The listing builds one solid part. Answer for the finished solid, in the listing's coordinates (mm). A direction names the side the tool comes from. Round coordinates to 2 decimals unless told otherwise and drop trailing zeros. Write each loop counter-clockwise with the first axis right and the second up, starting at its lowest first coordinate (ties: lowest second). Pieces come first, ordered by that corner, then holes.
Item 1: Find the intervals of material crossed by probe 1 along Y at (x, z) = (0, -4.3); probe 2 along X at (y, z) = (-2.6, -3.5); probe 3 along X at (y, z) = (2.5, 0.75), in increasing order.
Item 2: For a pull along X with two mould halves and no side action, classify faces 4 (the face through (0, 26, 5)), 5 (the face through (-6, 26, 0)), 6 (the face through (0, -2, -3.6)) as +X half, -X half, draft (parallel to the pull), parting line (faces both ways), or undercut.
Item 3: Find section B-B on x = 1.25. Give the vertices of the cut face in (y, z).
Item 4: Find section C-C on y = 43. Give the vertices of the cut face in (x, z), then the cut area to 3 significant figures.
Item 5: Find section A-A on z = 1. Give the vertices of the cut face in (x, y).
Item 6: A tool of negligible diameter and unlimited length cuts with its end or side. For faces 1 (the face through (0, 26, -5)), 2 (the face through (-2.7, 53.5, 0)), 3 (the face through (0, -2, 3.6)), from which of +Z, -Z, +X, -X, +Y, -Y can it reach the whole face along a straight path? Write none if from no direction.
```python
from build123d import *

# Parameters (mm, degrees)
SKETCH_1_W          = 12
SKETCH_1_H          = 10
SKETCH_1_W_2        = 6.2
SKETCH_1_H_2        = 6.2
EXTRUDE_1_DEPTH     = 54
EXTRUDE_START       = 54
SKETCH_1_3_W        = 12
SKETCH_1_3_H        = 10
SKETCH_1_3_W_2      = 6.2
SKETCH_1_3_H_2      = 6.2
SKETCH_1_3_W_3      = 5.4
SKETCH_1_3_H_3      = 5.4
EXTRUDE_2_DEPTH     = 1
SKETCH_3_W          = 12
SKETCH_3_H          = 10
SKETCH_3_W_2        = 7.2
SKETCH_3_H_2        = 7.2
EXTRUDE_3_DEPTH     = 3.4
SKETCH_2_R          = 0.3
CUT_EXTRUDE_1_DEPTH = 2
SKETCH_7_R          = 0.3
CUT_EXTRUDE_2_DEPTH = 56.244909268


with BuildPart() as part:
    # 草图1 → 凸台-拉伸1 (new body)
    with BuildSketch(Plane(origin=(0, 0, 0), x_dir=(1, 0, 0), z_dir=(0, 1, 0))):
        Rectangle(SKETCH_1_W, SKETCH_1_H)
        Rectangle(SKETCH_1_W_2, SKETCH_1_H_2, mode=Mode.SUBTRACT)
    extrude(amount=EXTRUDE_1_DEPTH)

    # 草图1<3> → 凸台-拉伸2 (add)
    # profile 1 of 2: a face of its own
    with BuildSketch(Plane(origin=(0, 0, 0), x_dir=(1, 0, 0), z_dir=(0, 1, 0)).offset(EXTRUDE_START)):
        Rectangle(SKETCH_1_3_W, SKETCH_1_3_H)
        Rectangle(SKETCH_1_3_W_2, SKETCH_1_3_H_2, mode=Mode.SUBTRACT)
    # profile 2 of 2: a face of its own
    with BuildSketch(Plane(origin=(0, 0, 0), x_dir=(1, 0, 0), z_dir=(0, 1, 0)).offset(EXTRUDE_START)):
        Rectangle(SKETCH_1_3_W_2, SKETCH_1_3_H_2)
        Rectangle(SKETCH_1_3_W_3, SKETCH_1_3_H_3, mode=Mode.SUBTRACT)
    extrude(amount=-EXTRUDE_2_DEPTH)

    # 草图3 → 凸台-拉伸3 (add)
    with BuildSketch(Plane.XZ):
        Rectangle(SKETCH_3_W, SKETCH_3_H)
        Rectangle(SKETCH_3_W_2, SKETCH_3_H_2, mode=Mode.SUBTRACT)
    extrude(amount=EXTRUDE_3_DEPTH)

    # 草图2 → 切除-拉伸1 (cut)
    with BuildSketch(Plane.XZ.offset(3.4)):
        with Locations(Location((-4.5, 3.5, 0), (0, 0, 270))):
            Circle(SKETCH_2_R)
        with Locations(Location((4.5, -3.5, 0), (0, 0, 270))):
            Circle(SKETCH_2_R)
        with Locations(Location((4.5, 3.5, 0), (0, 0, 270))):
            Circle(SKETCH_2_R)
        with Locations(Location((-4.5, -3.5, 0), (0, 0, 270))):
            Circle(SKETCH_2_R)
    extrude(amount=-CUT_EXTRUDE_1_DEPTH, mode=Mode.SUBTRACT)

    # 草图7 → 切除-拉伸2 (cut, through all)
    with BuildSketch(Plane(origin=(0, 0, -5), x_dir=(-1, 0, 0), z_dir=(0, 0, -1))):
        with Locations((0, 19)):
            Circle(SKETCH_7_R)
        with Locations((0, 25)):
            Circle(SKETCH_7_R)
        with Locations((0, 45)):
            Circle(SKETCH_7_R)
    extrude(amount=-CUT_EXTRUDE_2_DEPTH, mode=Mode.SUBTRACT)


solid = part.part
```
Check values:
1. probe 1: y = -3.4 to 18.7, 19.3 to 24.7, 25.3 to 44.7, 45.3 to 54
1. probe 2: x = -6 to -4.8, -4.2 to -3.6, 3.6 to 4.2, 4.8 to 6
1. probe 3: x = -6 to -3.1, 3.1 to 6
2. face 4: draft
2. face 5: -X half
2. face 6: undercut
3. outline: (-3.4, -5) - (54, -5) - (54, -2.7) - (53, -2.7) - (53, -3.1) - (0, -3.1) - (0, -3.6) - (-3.4, -3.6) - close; (-3.4, 3.6) - (0, 3.6) - (0, 3.1) - (53, 3.1) - (53, 2.7) - (54, 2.7) - (54, 5) - (-3.4, 5) - close
4. outline: (-6, -5) - (6, -5) - (6, 5) - (-6, 5) - close; hole (-3.1, -3.1) - (3.1, -3.1) - (3.1, 3.1) - (-3.1, 3.1) - close
4. area: 81.6 mm2
5. outline: (-6, -3.4) - (-3.6, -3.4) - (-3.6, 0) - (-3.1, 0) - (-3.1, 53) - (-2.7, 53) - (-2.7, 54) - (-6, 54) - close; (2.7, 53) - (3.1, 53) - (3.1, 0) - (3.6, 0) - (3.6, -3.4) - (6, -3.4) - (6, 54) - (2.7, 54) - close
6. face 1: -Z, +X, -X, +Y, -Y
6. face 2: +Y, -Y
6. face 3: -Y
